from build123d import *

# Parameters (mm, degrees)
Y_KSEKLIK_EKSTR_ZYON1_DEPTH = 2
Y_KSEKLIK_EKSTR_ZYON2_DEPTH = 5
IZIM3_W                     = 71.3
IZIM3_H                     = 24.4
KES_EKSTR_ZYON1_DEPTH       = 5
IZIM4_R                     = 2.5
IZIM4_R_2                   = 1.5
Y_KSEKLIK_EKSTR_ZYON3_DEPTH = 5.4


with BuildPart() as part:
    # Çizim1 → Yükseklik-Ekstrüzyon1 (new body)
    with BuildSketch(Plane(origin=(0, 0, 0), x_dir=(1, 0, 0), z_dir=(0, 1, 0))):
        with BuildLine():
            Line((10, 0), (90, 0))
            ThreePointArc((90, 0), (97.071067812, 2.928932188), (100, 10))
            Line((100, 10), (100, 50))
            ThreePointArc((100, 50), (97.071067812, 57.071067812), (90, 60))
            Line((90, 60), (10, 60))
            ThreePointArc((10, 60), (2.928932188, 57.071067812), (0, 50))
            Line((0, 50), (0, 10))
            ThreePointArc((0, 10), (2.928932188, 2.928932188), (10, 0))
        make_face()
    extrude(amount=Y_KSEKLIK_EKSTR_ZYON1_DEPTH)

    # Çizim2 → Yükseklik-Ekstrüzyon2 (add)
    with BuildSketch(Plane(origin=(0, 2, 0), x_dir=(1, 0, 0), z_dir=(0, 1, 0))):
        Polygon((12, 2), (88, 2), (98, 12), (98, 48), (88, 58), (12, 58), (2, 48), (2, 12), align=None)
        Polygon((4, 46), (4, 14), (14, 4), (86, 4), (96, 14), (96, 46), (86, 56), (14, 56), align=None, mode=Mode.SUBTRACT)
    extrude(amount=Y_KSEKLIK_EKSTR_ZYON2_DEPTH)

    # Çizim3 → Kes-Ekstrüzyon1 (cut)
    with BuildSketch(Plane(origin=(0, 2, 0), x_dir=(1, 0, 0), z_dir=(0, 1, 0))):
        with Locations((50, 30)):
            Rectangle(IZIM3_W, IZIM3_H)
    extrude(amount=-KES_EKSTR_ZYON1_DEPTH, mode=Mode.SUBTRACT)

    # Çizim4 → Yükseklik-Ekstrüzyon3 (add)
    # profile 1 of 4: a face of its own
    with BuildSketch(Plane(origin=(0, 2, 0), x_dir=(1, 0, 0), z_dir=(0, 1, 0))):
        with Locations(Location((12.5, 45.5, 0), (0, 0, 90))):
            Circle(IZIM4_R)
        with Locations(Location((12.5, 45.5, 0), (0, 0, 90))):
            Circle(IZIM4_R_2, mode=Mode.SUBTRACT)
    # profile 2 of 4: a face of its own
    with BuildSketch(Plane(origin=(0, 2, 0), x_dir=(1, 0, 0), z_dir=(0, 1, 0))):
        with Locations(Location((87.5, 45.5, 0), (0, 0, 90))):
            Circle(IZIM4_R)
        with Locations(Location((87.5, 45.5, 0), (0, 0, 90))):
            Circle(IZIM4_R_2, mode=Mode.SUBTRACT)
    # profile 3 of 4: a face of its own
    with BuildSketch(Plane(origin=(0, 2, 0), x_dir=(1, 0, 0), z_dir=(0, 1, 0))):
        with Locations(Location((87.5, 14.5, 0), (0, 0, 90))):
            Circle(IZIM4_R)
        with Locations(Location((87.5, 14.5, 0), (0, 0, 90))):
            Circle(IZIM4_R_2, mode=Mode.SUBTRACT)
    # profile 4 of 4: a face of its own
    with BuildSketch(Plane(origin=(0, 2, 0), x_dir=(1, 0, 0), z_dir=(0, 1, 0))):
        with Locations(Location((12.5, 14.5, 0), (0, 0, 90))):
            Circle(IZIM4_R)
        with Locations(Location((12.5, 14.5, 0), (0, 0, 90))):
            Circle(IZIM4_R_2, mode=Mode.SUBTRACT)
    extrude(amount=Y_KSEKLIK_EKSTR_ZYON3_DEPTH)


solid = part.part
Source: CAD feature listing. Evaluate the final solid. Frame: model axes, mm. A direction names the side the tool comes from. Round coordinates to 2 decimals unless told otherwise and drop trailing zeros. Loops run counter-clockwise (first coordinate to the right, second up) from the corner with the lowest first, then second, coordinate; pieces in that order, holes last. Notation, with made-up numbers: (-29.75, -12) -> (-17.75, -12) arc R16 cw to (-17.75, -2) -> close; hole circle Ø9 at (55.25, 20). An arc over 180 degrees is marked (long way). Answer as a JSON object with one key per item and string values. Group by question number.
Q1. Mould query, pull axis X, two halves, no side actions, for faces 1 (the flat face through (14.35, 1, -30)), 2 (the flat face through (43, 7, -57)), 3 (the cylindrical face through (2.85, 0.99, -3.01)). Classes: pulls with the +X half, pulls with the -X half, needs draft (parallel to the pull), parting line crosses it, or undercut.
Q2. Section query C-C (x = 29). Output: boundary loops of the cut face in (y, z), plus the area to 3 significant figures.
Q3. Ray query, line 1 (X direction, y = 3.9, z = -14.5); line 2 (Z direction, x = 72, y = 6); line 3 (X direction, y = 3, z = -20.5). Return the intervals inside material, ascending. Write a range as from..to.
Q4. Section query A-A (y = 3). State how many separate pieces and enclosed holes the cut face has, plus the area to 3 significant figures.
Q5. Access query for faces 4 (the flat face through (89, 7.4, -47)), 5 (the flat face through (93, 4, -53)), 6 (the cylindrical face through (85.02, 4.66, -45.17)), 7 (the flat face through (98, 4, -30)). Directions: +Z, -Z, +X, -X, +Y, -Y. A direction counts if a zero-diameter tool reaches every point of the face in a straight line with its end or side. Return the directions, or none.
Q6. Section query B-B (z = -39). Output: boundary loops of the cut face in (x, y), plus the area to 3 significant figures.
Q7. Contact query for flat-ended pins moving along their axis: P1, Ø4, axis at x = 32, y = 5.5, coming from the +Z side; P2, Ø2, axis at x = 72.5, z = -46, coming from the -Y side; P3, Ø1.5, axis at x = 57.5, y = 5, coming from the -Z side; P4, Ø0.9, axis at x = 12, z = -14, coming from the +Y side. Output: stop coordinate, or through.
Completed:
{
 "1": {"face 1": "undercut", "face 2": "needs draft", "face 3": "pulls with the -X half"},
 "2": {"outline": "(0, -60) -> (2, -60) -> (2, -58) -> (7, -58) -> (7, -56) -> (2, -56) -> (2, -42.2) -> (0, -42.2) -> close; (0, -17.8) -> (2, -17.8) -> (2, -4) -> (7, -4) -> (7, -2) -> (2, -2) -> (2, 0) -> (0, 0) -> close", "area": "91.2 mm²"},
 "3": {"line 1": "2..4, 10..11, 14..15, 85..86, 89..90, 96..98", "line 2": "-58..-56, -4..-2", "line 3": "2..4, 96..98"},
 "4": {"separate pieces": "5", "enclosed holes": "5", "area": "642 mm²"},
 "5": {"face 4": "+Z, -Z, +X, -X, +Y", "face 5": "-Z, +X, +Y", "face 6": "+Y", "face 7": "+Z, -Z, +X, +Y"},
 "6": {"outline": "(0, 0) -> (14.35, 0) -> (14.35, 2) -> (4, 2) -> (4, 7) -> (2, 7) -> (2, 2) -> (0, 2) -> close; (85.65, 0) -> (100, 0) -> (100, 2) -> (98, 2) -> (98, 7) -> (96, 7) -> (96, 2) -> (85.65, 2) -> close", "area": "77.4 mm²"},
 "7": {"P1": "z = -2", "P2": "y = 0", "P3": "z = -58", "P4": "y = 2"}
}
